Source: three-view drawing plus pictorial views. Frame: mm from the lowest corner of the part. A direction names the side the tool comes from. Give positions to 0.01 mm unless a question says otherwise; leave off trailing zeros. Write each loop counter-clockwise with the first axis right and the second up, starting at its lowest first coordinate (ties: lowest second). Pieces come first, ordered by that corner, then holes.
Q1. Cut plane A-A on y = 39. Return the cut outline in (x, z), plus the area to 3 significant figures.
Q2. Cut plane B-B on x = 43. Return the cut outline in (y, z), plus the area to 3 significant figures.
Q3. Reachability of the marked faces 1, 2, 3 and 4 from +Z, -Z, +X, -X, +Y, -Y: full face, straight path, thin tool, end or side. Return the list, or none.
Q4. Cut plane C-C on z = 27.5. Return the cut outline in (x, y).
Q5. Line query: L1, parallel to X at y = 12.5, z = 17.5; L2, parallel to Y at x = 47.5, z = 2.5; L3, parallel to Y at x = 8, z = 34. Output: solid intervals per line, ascending.
Q6. Pin query (flat end, axial travel): pin 1 (8 mm diameter, centred on y = 9, z = 5, fed in from +X); pin 2 (1.5 mm diameter, centred on x = 12.5, y = 25, fed in from +Z); pin 3 (13 mm diameter, centred on x = 22, z = 22, fed in from -Y). Return the tip coordinate at first contact, or that it passes through.
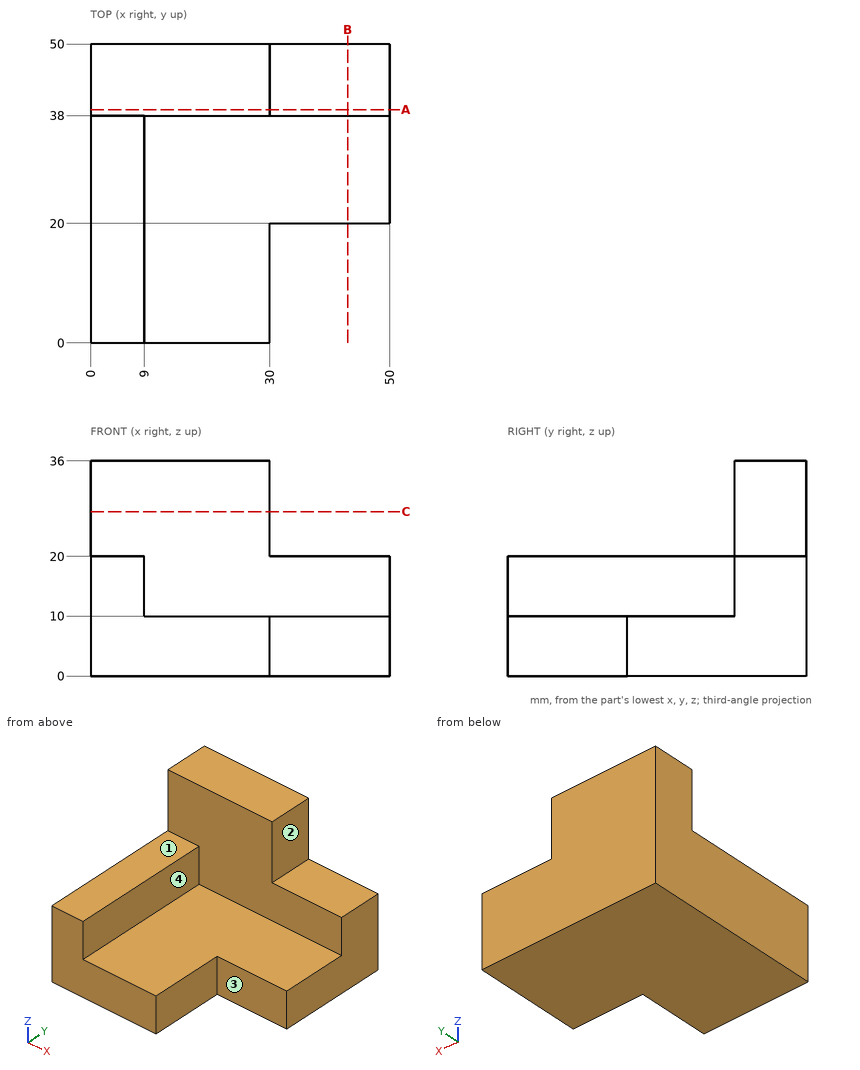
Data:
1. outline: (0, 0) - (50, 0) - (50, 20) - (30, 20) - (30, 36) - (0, 36) - close
1. area: 1,480 mm2
2. outline: (20, 0) - (50, 0) - (50, 20) - (38, 20) - (38, 10) - (20, 10) - close
2. area: 420 mm2
3. face 1: +Z, +X, -X, -Y
3. face 2: +Z, +X, +Y, -Y
3. face 3: +Z, -Z, +X, -Y
3. face 4: +Z, +X, -Y
4. outline: (0, 38) - (30, 38) - (30, 50) - (0, 50) - close
5. L1: x = 0 to 9
5. L2: y = 20 to 50
5. L3: y = 38 to 50
6. pin 1: stops at x = 30
6. pin 2: stops at z = 10
6. pin 3: stops at y = 38
